Read the model definition and answer for the solid it produces. Units are mm, in the model's axes. Coordinates: 2 decimals unless noted, no trailing zeros. Write each loop counter-clockwise with the first axis right and the second up, starting at its lowest first coordinate (ties: lowest second). Pieces come first, ordered by that corner, then holes. Notation, with made-up numbers: (-13.5, 76) -> (40.5, 76) arc R22 ccw to (40.5, 105) -> close; hole circle Ø7 at (-35.5, 27). An arc over 180 degrees is marked (long way). Answer as a JSON object with one key per item and string values. Group by question number.
(1) Find section C-C (y = 217). Give the vertices of the cut face in (x, z), then the cut area to 3 significant figures.
(2) Find section A-A (x = 0). Give the vertices of the cut face in (y, z), then the cut area to 3 significant figures.
(3) Straight lines are drawn through the part: L1, parallel to Y at x = 1.75, z = 220; L2, parallel to Y at x = 0, z = 238; L3, parallel to Z at x = -0.5, y = 42. For each, find the intervals that lie inside material, in ascending order.
(4) Flat-ended cylindrical pins translate along their axes: P1, Ø3, axis at x = -1.5, y = 264, coming from the +Z side; P2, Ø4, axis at x = 2.5, y = 89.5, coming from the -Z side; P3, Ø1.5, axis at x = -3, z = 128, coming from the -Y side. Find the tip coordinate at first contact, or state that the pin passes through.
(5) Find section B-B (z = 378). Give the vertices of the cut face in (x, y), then the cut area to 3 significant figures.
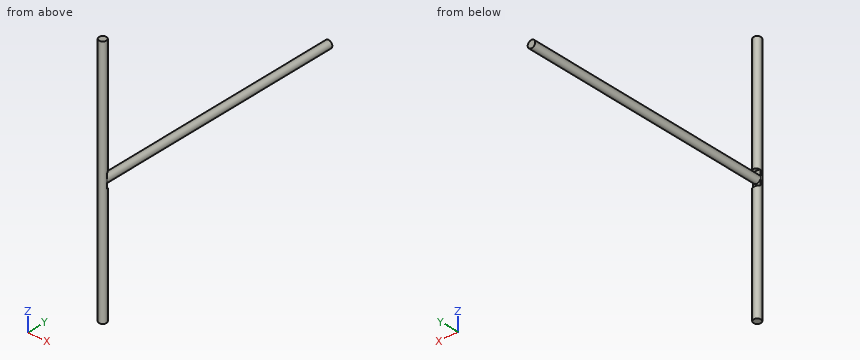
from build123d import *

# Parameters (mm, degrees)
SKETCH1_R           = 7.5
BOSS_EXTRUDE1_DEPTH = 500
SKETCH2_R           = 16
CUT_EXTRUDE1_DEPTH  = 15
SKETCH4_R           = 7.5
BOSS_EXTRUDE2_DEPTH = 499


with BuildPart() as part:
    # Sketch1 → Boss-Extrude1 (new body)
    with BuildSketch(Plane.XY):
        Circle(SKETCH1_R)
    extrude(amount=BOSS_EXTRUDE1_DEPTH)

    # Sketch2 → Cut-Extrude1 (cut)
    with BuildSketch(Plane(origin=(0, 16, 0), x_dir=(1, 0, 0), z_dir=(0, 1, 0))):
        with Locations((0, -250.362407272)):
            Circle(SKETCH2_R)
    extrude(amount=-CUT_EXTRUDE1_DEPTH, mode=Mode.SUBTRACT)

    # Sketch4 → Boss-Extrude2 (add)
    with BuildSketch(Plane(origin=(0, 1, 0), x_dir=(1, 0, 0), z_dir=(0, 1, 0))):
        with Locations((0, -250.362407272)):
            Circle(SKETCH4_R)
    extrude(amount=BOSS_EXTRUDE2_DEPTH)


solid = part.part
Results below:
{
 "1": {"outline": "circle Ø15 at (0, 250.36)", "area": "177 mm2"},
 "2": {"outline": "(-7.5, 0) -> (7.5, 0) -> (7.5, 234.36) -> (1, 234.36) -> (1, 242.86) -> (500, 242.86) -> (500, 257.86) -> (1, 257.86) -> (1, 266.36) -> (7.5, 266.36) -> (7.5, 500) -> (-7.5, 500) -> close", "area": "14,800 mm2"},
 "3": {"L1": "y = -7.29 to 7.29", "L2": "y = -7.5 to 1", "L3": "z = 242.88 to 257.85"},
 "4": {"P1": "stops at z = 257.86", "P2": "stops at z = 242.88", "P3": "stops at y = -7.15"},
 "5": {"outline": "circle Ø15 at (0, 0)", "area": "177 mm2"}
}
